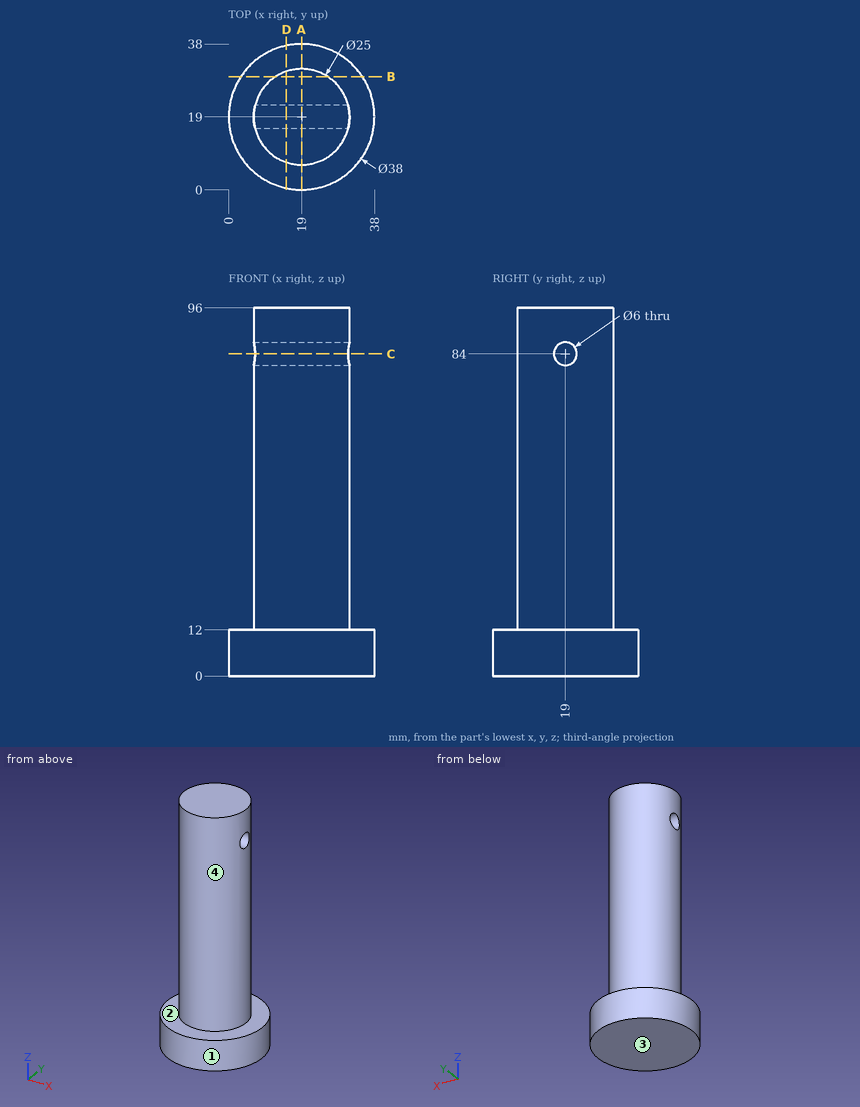
Job drawing, mm, ordinate dimensions from the low corner. One solid piece. A direction names the side the tool comes from. Coordinates: 2 decimals unless noted, no trailing zeros. Write each loop counter-clockwise with the first axis right and the second up, starting at its lowest first coordinate (ties: lowest second). Pieces come first, ordered by that corner, then holes. Notation, with made-up numbers: (78.25, -3) -> (109.25, -3) arc R26 cw to (109.25, 16) -> close; hole circle Ø4 at (-15.75, 85.25). An arc over 180 degrees is marked (long way). Use CSV: the item, a comma, the result in double quotes. Start each with the question number.
Item 1: Wall check: probe 1 along Z at (x, y) = (14, 19); probe 2 along Z at (x, y) = (8, 7.5); probe 3 along Y at (x, z) = (19.5, 84). Give the ranges that are in metal, low to high.
Item 2: Drop flat-ended pins along their axis: P1, Ø10, axis at x = 34, z = 41.5, coming from the -Y side; P2, Ø8, axis at x = 22.5, z = 32.5, coming from the +Y side; P3, Ø3, axis at y = 30.5, z = 22, coming from the +X side. Give the stop position or say it passes through.
Item 3: Tool access for the marked faces 3 and 4: list every direction of +Z, -Z, +X, -X, +Y, -Y with a clear straight run to the whole face (end or side of a thin tool).
Item 4: Band-saw the part on D-D, the plane x = 15. Write the cut outline in (y, z), plus the area to 3 significant figures.
Item 5: Two-plate mould, pull along Y, no slides. Class the marked faces 1 and 2: +Y half, -Y half, draft (parallel to the pull), parting line (faces both ways), or undercut.
Item 6: Band-saw the part on B-B, the plane y = 29.5. Write the cut outline in (x, z).
Item 7: Band-saw the part on C-C, the plane z = 84. Write the cut outline in (x, y).
Item 8: Band-saw the part on A-A, the plane x = 19. Write the cut outline in (y, z), plus the area to 3 significant figures.
Response values:
1,probe 1,"z = 0 to 81, 87 to 96"
1,probe 2,"z = 0 to 12"
1,probe 3,"y = 6.51 to 16, 22 to 31.49"
2,P1,"stops at y = 11.5"
2,P2,"stops at y = 31.5"
2,P3,"stops at x = 26.5"
3,face 3,"-Z, +X, -X, +Y, -Y"
3,face 4,"+Z"
4,outline,"(0.43, 0) -> (37.57, 0) -> (37.57, 12) -> (30.84, 12) -> (30.84, 96) -> (7.16, 96) -> (7.16, 12) -> (0.43, 12) -> close; hole circle Ø6 at (19, 84)"
4,area,"2,410 mm2"
5,face 1,"parting line"
5,face 2,"draft"
6,outline,"(3.16, 0) -> (34.84, 0) -> (34.84, 12) -> (25.78, 12) -> (25.78, 96) -> (12.22, 96) -> (12.22, 12) -> (3.16, 12) -> close"
7,outline,"(6.87, 16) arc R12.5 ccw to (31.13, 16) -> close; (6.87, 22) -> (31.13, 22) arc R12.5 ccw to start"
8,outline,"(0, 0) -> (38, 0) -> (38, 12) -> (31.5, 12) -> (31.5, 96) -> (6.5, 96) -> (6.5, 12) -> (0, 12) -> close; hole circle Ø6 at (19, 84)"
8,area,"2,530 mm2"
